from build123d import *

# Parameters (mm, degrees)
F0_W     = 1040
F0_H     = 470
F1_DEPTH = 32
F2_W     = 800
F2_H     = 260
F3_DEPTH = 32.001


with BuildPart() as f1:
    # F0 (on Top) → F1 (new body)
    with BuildSketch(Plane.XY):
        Rectangle(F0_W, F0_H)
    extrude(amount=F1_DEPTH)

    # F2 (on Top) → F3 (cut, through all)
    with BuildSketch(Plane.XY):
        with Locations((0, -25)):
            Rectangle(F2_W, F2_H)
    extrude(amount=F3_DEPTH, mode=Mode.SUBTRACT)


solid = f1.part
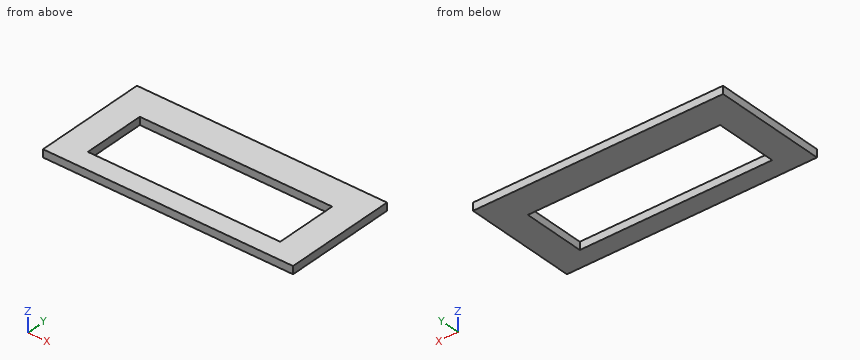
Could you check a few things on this model? Use its own coordinates, in mm. Give positions to 0.01 mm unless a question says otherwise; leave off trailing zeros. Loops run counter-clockwise (first coordinate to the right, second up) from the corner with the lowest first, then second, coordinate; pieces in that order, holes last. Notation, with made-up numbers: (21.25, 33) -> (68.25, 33) arc R28 cw to (68.25, 66) -> close; hole circle Ø8 at (-35, 18.25). An arc over 180 degrees is marked (long way). Return JSON: item names as keys, results as strings.
Item 1: If we section it at C-C on z = 19.5: List the corners of the cut face in (x, y) for me, plus the area to 3 significant figures.
Geometry results:
{"outline": "(-520, -235) -> (520, -235) -> (520, 235) -> (-520, 235) -> close; hole (-400, -155) -> (400, -155) -> (400, 105) -> (-400, 105) -> close", "area": "281,000 mm²"}
Item 2: If we section it at A-A on x = 0: List the corners of the cut face in (y, z) for me.
Geometry results:
{"outline": "(-235, 0) -> (-155, 0) -> (-155, 32) -> (-235, 32) -> close; (105, 0) -> (235, 0) -> (235, 32) -> (105, 32) -> close"}
Item 3: I need wall thicknesses on L1, parallel to X at y = 24, z = 5.5; L2, parallel to Y at x = 34.5, z = 26. Which ranges of each line are inside material? Lowest first, please. Write a range as from..to.
Geometry results:
{"L1": "x = -520..-400, 400..520", "L2": "y = -235..-155, 105..235"}
Item 4: If we section it at B-B on y = 94.5: List the corners of the cut face in (x, z) for me.
Geometry results:
{"outline": "(-520, 0) -> (-400, 0) -> (-400, 32) -> (-520, 32) -> close; (400, 0) -> (520, 0) -> (520, 32) -> (400, 32) -> close"}
